```python
from build123d import *

# Parameters (mm, degrees)
SKETCH1_R           = 9.5
SKETCH1_R_2         = 2
BOSS_EXTRUDE2_DEPTH = 5
SKETCH2_R           = 2
CUT_EXTRUDE1_DEPTH  = 43.5


with BuildPart() as part:
    # Sketch1 → Boss-Extrude2 (new, symmetric)
    with BuildSketch(Plane.XY):
        with BuildLine():
            Line((0, 0), (-25, 0))
            Line((-25, 0), (-79.465738474, 79.800827522))
            ThreePointArc((-79.465738474, 79.800827522), (-81.213991187, 110.724247098), (-54.687026413, 126.712818196))
            Line((-54.687026413, 126.712818196), (122.946920772, 126.712818196))
            Line((122.946920772, 126.712818196), (130, 86.712818196))
            Line((130, 86.712818196), (-16.822273347, 86.712818196))
            ThreePointArc((-16.822273347, 86.712818196), (-25.664594939, 81.383294497), (-25.081844034, 71.075487971))
            Line((-25.081844034, 71.075487971), (0, 34.32666264))
            Line((0, 34.32666264), (0, 0))
        make_face()
        with Locations((-54.687026413, 96.712818196)):
            Circle(SKETCH1_R, mode=Mode.SUBTRACT)
        with Locations((118.092164461, 116.712818196)):
            Circle(SKETCH1_R_2, mode=Mode.SUBTRACT)
        with Locations((123.092164461, 96.712818196)):
            Circle(SKETCH1_R_2, mode=Mode.SUBTRACT)
        with BuildLine():
            Line((87.602603423, 114.955476372), (115.489324713, 101.027318395))
            ThreePointArc((115.489324713, 101.027318395), (117.068751792, 97.654829908), (114.148854559, 95.343451825))
            Line((114.148854559, 95.343451825), (67.87894889, 95.343451825))
            ThreePointArc((67.87894889, 95.343451825), (65.035223605, 97.387822973), (66.067251604, 100.734634156))
            Line((66.067251604, 100.734634156), (84.450435982, 114.662792133))
            ThreePointArc((84.450435982, 114.662792133), (85.984771107, 115.258760656), (87.602603423, 114.955476372))
        make_face(mode=Mode.SUBTRACT)
        with BuildLine():
            Line((-0.491145104, 115.057882008), (27.475527786, 101.02482381))
            ThreePointArc((27.475527786, 101.02482381), (29.049331009, 97.652118315), (26.130074601, 95.343451825))
            Line((26.130074601, 95.343451825), (-20.139831067, 95.343451825))
            ThreePointArc((-20.139831067, 95.343451825), (-22.980812237, 97.379695636), (-21.965173191, 100.724234497))
            Line((-21.965173191, 100.724234497), (-3.661940413, 114.757292695))
            ThreePointArc((-3.661940413, 114.757292695), (-2.119726939, 115.363119834), (-0.491145104, 115.057882008))
        make_face(mode=Mode.SUBTRACT)
        with BuildLine():
            Line((26.031042482, 117.478697139), (61.470853651, 117.478697139))
            ThreePointArc((61.470853651, 117.478697139), (64.314578937, 115.434325991), (63.282550938, 112.087514808))
            Line((63.282550938, 112.087514808), (49.162800513, 101.389579648))
            ThreePointArc((49.162800513, 101.389579648), (47.625690916, 100.793354809), (46.005650041, 101.099389994))
            Line((46.005650041, 101.099389994), (24.685589296, 111.797325153))
            ThreePointArc((24.685589296, 111.797325153), (23.111786073, 115.170030649), (26.031042482, 117.478697139))
        make_face(mode=Mode.SUBTRACT)
        with BuildLine():
            Line((-44.320136127, 47.300576318), (-34.048206361, 32.250592263))
            ThreePointArc((-34.048206361, 32.250592263), (-32.202518151, 31.009156908), (-30.009288975, 31.379929737))
            Line((-30.009288975, 31.379929737), (-16.865487004, 39.388981395))
            ThreePointArc((-16.865487004, 39.388981395), (-15.450916476, 42.332556513), (-17.56266475, 44.823773781))
            Line((-17.56266475, 44.823773781), (-40.978396488, 51.864706177))
            ThreePointArc((-40.978396488, 51.864706177), (-44.262816837, 50.76404185), (-44.320136127, 47.300576318))
        make_face(mode=Mode.SUBTRACT)
    extrude(amount=BOSS_EXTRUDE2_DEPTH, both=True)

    # Sketch2 → Cut-Extrude1 (cut, symmetric)
    with BuildSketch(Plane(origin=(0, 0, 0), x_dir=(0, 0, -1), z_dir=(1, 0, 0))):
        with Locations(Location((0, 5, 0), (0, 0, 90))):
            Circle(SKETCH2_R)
        with Locations(Location((0, 20, 0), (0, 0, 90))):
            Circle(SKETCH2_R)
    extrude(amount=CUT_EXTRUDE1_DEPTH, both=True, mode=Mode.SUBTRACT)


solid = part.part
```
CAD build for the part. Positions are in the model's coordinates, mm. A direction names the side the tool comes from. Round coordinates to 2 decimals unless told otherwise and drop trailing zeros. Write each loop counter-clockwise with the first axis right and the second up, starting at its lowest first coordinate (ties: lowest second). Pieces come first, ordered by that corner, then holes. Notation, with made-up numbers: (-30.75, 25) -> (-15.75, 25) arc R18 cw to (-15.75, 40) -> close; hole circle Ø4 at (48.5, 0.25). An arc over 180 degrees is marked (long way). Answer in a Markdown table with one row per item. Add a question column.
Item 1: Mould opens along Y. For faces 1 (the face through (-12, 0, 0)), 2 (the face through (125, 97.31, -0.07)), 3 (the face through (33, 126.713, 0)) say: pulls with the +Y half, pulls with the -Y half, needs draft (parallel to the pull), parting line crosses it, or undercut.
Item 2: Saw through at D-D, the plane z = 0. Count the separate pieces of the cut face and the enclosed holes in it, then the cut area to 3 significant figures.
Item 3: Saw through at B-B, the plane x = 20. Write the cut outline in (y, z), then the cut area to 3 significant figures.
Item 4: Drill centre lines: line 1 (Z direction, x = -16, y = 5); line 2 (X direction, y = 98, z = 3.5); line 3 (X direction, y = 106.5, z = 3.25). Where is each one in solid material? Low to high. Write a range as from..to.
Item 5: Saw through at A-A, the plane y = 109. Write the cut outline in (x, z), then the cut area to 3 significant figures.
Item 6: Which spindle directions (+Z, -Z, +X, -X, +Y, -Y) get a long thin tool onto all of the face, cutting with end or side? Do faces 4 (the face through (64.3, 115.48, 0.07)), 5 (the face through (-51.85, 39.34, 0.07)). Say none if no direction does.
Item 7: Saw through at C-C, the plane y = 20. Write the cut outline in (x, z).
Item 8: Drop flat-ended pins along their axis: pin 1 Ø3.5 at (x, y) = (118.09, 116.71) entering from +Z; pin 2 Ø1 at (y, z) = (57.5, 1) entering from -X; pin 3 Ø3 at (y, z) = (25.5, 2) entering from +X; pin 4 Ø2 at (y, z) = (17, 2) entering from -X. Give the stop position or say it passes through.
Findings below:
| question | item | result |
|---|---|---|
| 1 | face 1 | pulls with the -Y half |
| 1 | face 2 | undercut |
| 1 | face 3 | pulls with the +Y half |
| 2 | separate pieces | 3 |
| 2 | enclosed holes | 7 |
| 2 | area | 9,450 mm^2 |
| 3 | outline | (86.71, -5) -> (95.34, -5) -> (95.34, 5) -> (86.71, 5) -> close; (104.78, -5) -> (126.71, -5) -> (126.71, 5) -> (104.78, 5) -> close |
| 3 | area | 306 mm^2 |
| 4 | line 1 | z = -5..-2, 2..5 |
| 4 | line 2 | x = -84.66..-64.1, -45.27..-23.12, 29.11..64.9, 117.13..121.56, 124.62..128.01 |
| 4 | line 3 | x = -83.05..-14.43, 16.56..35.24, 55.91..73.68, 104.53..126.51 |
| 5 | outline | (-82.06, -5) -> (-11.17, -5) -> (-11.17, 5) -> (-82.06, 5) -> close; (11.58, -5) -> (30.26, -5) -> (30.26, 5) -> (11.58, 5) -> close; (59.21, -5) -> (76.98, -5) -> (76.98, 5) -> (59.21, 5) -> close; (99.53, -5) -> (126.07, -5) -> (126.07, 5) -> (99.53, 5) -> close |
| 5 | area | 1,340 mm^2 |
| 6 | face 4 | +Z, -Z |
| 6 | face 5 | +Z, -Z, -X, -Y |
| 7 | outline | (-38.65, -5) -> (0, -5) -> (0, -2) -> (-38.65, -2) -> close; (-38.65, 2) -> (0, 2) -> (0, 5) -> (-38.65, 5) -> close |
| 8 | pin 1 | passes through |
| 8 | pin 2 | stops at x = -64.59 |
| 8 | pin 3 | stops at x = 0 |
| 8 | pin 4 | stops at x = -37.29 |
